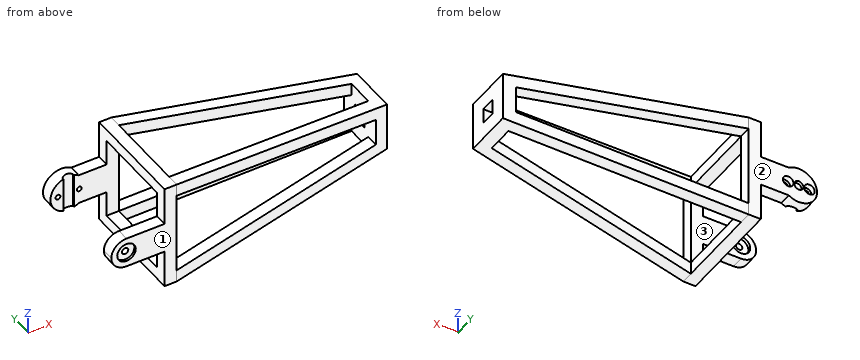
```python
from build123d import *

# Parameters (mm, degrees)
SZKIC1_W                        = 43
SZKIC1_H                        = 20
SZKIC1_R                        = 2.1
DODANIE_WYCI_GNI_CIE1_DEPTH     = 8
SZKIC2_R                        = 6.1
WYTNIJ_WYCI_GNI_CIE1_DEPTH      = 2
WYTNIJ_WYCI_GNI_CIE2_START      = -1.5
SZKIC3_R                        = 6.1
WYTNIJ_WYCI_GNI_CIE2_DEPTH      = 1.5
SZKIC4_W                        = 8
SZKIC4_H                        = 20
DODANIE_WYCI_GNI_CIE2_DEPTH     = 54
ZAOKR_GLENIE1_R                 = 10
DODANIE_WYCI_GNI_CIE3_DEPTH     = 8
WYTNIJ_WYCI_GNI_CIE3_REACH      = 80.313
SZKIC6_R                        = 1.6
SZKIC7_R                        = 3.5
WYTNIJ_WYCI_GNI_CIE4_DEPTH      = 3.5
WYTNIJ_WYCI_GNI_CIE5_REACH      = 83.025
WYTNIJ_WYCI_GNI_CIE5_END_RADIUS = 12
SZKIC10_R                       = 3
WYTNIJ_WYCI_GNI_CIE6_DEPTH      = 2
SZKIC13_W                       = 25
SZKIC13_H                       = 70
DODANIE_WYCI_GNI_CIE4_DEPTH     = 8
WYTNIJ_WYCI_GNI_CIE7_REACH      = 88.568
SZKIC14_W                       = 54
SZKIC14_H                       = 54
DODANIE_WYCI_GNI_CIE5_DEPTH     = 70
WYTNIJ_WYCI_GNI_CIE9_DEPTH      = 209.060087508
WYTNIJ_WYCI_GNI_CIE10_REACH     = 212.119
SZKIC20_W                       = 10
SZKIC20_H                       = 10


with BuildPart() as part:
    # Szkic1 → Dodanie-wyciągnięcie1 (new body)
    with BuildSketch(Plane(origin=(0, 0, 0), x_dir=(1, 0, 0), z_dir=(0, 1, 0))):
        with Locations((11.5, 0)):
            Rectangle(SZKIC1_W, SZKIC1_H)
        with Locations(Location((0, 0, 0), (0, 0, 270))):
            Circle(SZKIC1_R, mode=Mode.SUBTRACT)
    extrude(amount=DODANIE_WYCI_GNI_CIE1_DEPTH)

    # Szkic2 → Wytnij-wyciągnięcie1 (cut)
    with BuildSketch(Plane(origin=(0, 8, 0), x_dir=(1, 0, 0), z_dir=(0, 1, 0))):
        with Locations(Location((0, 0, 0), (0, 0, 270))):
            Circle(SZKIC2_R)
    extrude(amount=-WYTNIJ_WYCI_GNI_CIE1_DEPTH, mode=Mode.SUBTRACT)

    # Szkic3 → Wytnij-wyciągnięcie2 (cut)
    with BuildSketch(Plane.XZ.offset(WYTNIJ_WYCI_GNI_CIE2_START)):
        with Locations(Location((0, 0, 0), (0, 0, 90))):
            Circle(SZKIC3_R)
    extrude(amount=WYTNIJ_WYCI_GNI_CIE2_DEPTH, mode=Mode.SUBTRACT)

    # Szkic4 → Dodanie-wyciągnięcie2 (add)
    with BuildSketch(Plane(origin=(0, 8, 0), x_dir=(1, 0, 0), z_dir=(0, 1, 0))):
        with Locations((29, 0)):
            Rectangle(SZKIC4_W, SZKIC4_H)
    extrude(amount=DODANIE_WYCI_GNI_CIE2_DEPTH)

    # Zaokrąglenie1
    zaokr_glenie1_edges = [part.edges().sort_by_distance(p)[0] for p in [
        (-10, 4, -10),
        (-10, 4, 10),
    ]]
    fillet(zaokr_glenie1_edges, radius=ZAOKR_GLENIE1_R - 0.0001)  # a hair under: the kernel refuses the full size

    # Szkic5 → Dodanie-wyciągnięcie3 (add)
    with BuildSketch(Plane(origin=(0, 62, 0), x_dir=(1, 0, 0), z_dir=(0, 1, 0))):
        with BuildLine():
            Line((33, -10), (33, 10))
            Line((33, 10), (6.633249581, 10))
            ThreePointArc((6.633249581, 10), (-12, 0), (6.633249581, -10))
            Line((6.633249581, -10), (33, -10))
        make_face()
    extrude(amount=DODANIE_WYCI_GNI_CIE3_DEPTH)

    # Szkic6 → Wytnij-wyciągnięcie3 (cut, up to next)
    with BuildSketch(Plane(origin=(0, 70, 0), x_dir=(1, 0, 0), z_dir=(0, 1, 0)), mode=Mode.PRIVATE) as wytnij_wyci_gni_cie3_sk1:
        with Locations(Location((-7, 0, 0), (0, 0, 270))):
            Circle(SZKIC6_R)
    wytnij_wyci_gni_cie3_tool1 = extrude(wytnij_wyci_gni_cie3_sk1.sketch, amount=-WYTNIJ_WYCI_GNI_CIE3_REACH, mode=Mode.PRIVATE) & part.part
    # Szkic6 → Wytnij-wyciągnięcie3 (cut, up to next)
    with BuildSketch(Plane(origin=(0, 70, 0), x_dir=(1, 0, 0), z_dir=(0, 1, 0)), mode=Mode.PRIVATE) as wytnij_wyci_gni_cie3_sk2:
        with Locations(Location((7, 0, 0), (0, 0, 270))):
            Circle(SZKIC6_R)
    wytnij_wyci_gni_cie3_tool2 = extrude(wytnij_wyci_gni_cie3_sk2.sketch, amount=-WYTNIJ_WYCI_GNI_CIE3_REACH, mode=Mode.PRIVATE) & part.part
    add(wytnij_wyci_gni_cie3_tool1.solids().sort_by_distance((-7, 70, 0))[0], mode=Mode.SUBTRACT)
    add(wytnij_wyci_gni_cie3_tool2.solids().sort_by_distance((7, 70, 0))[0], mode=Mode.SUBTRACT)

    # Szkic7 → Wytnij-wyciągnięcie4 (cut)
    with BuildSketch(Plane(origin=(0, 70, 0), x_dir=(1, 0, 0), z_dir=(0, 1, 0))):
        with Locations(Location((7, 0, 0), (0, 0, 270))):
            Circle(SZKIC7_R)
        with Locations(Location((-7, 0, 0), (0, 0, 270))):
            Circle(SZKIC7_R)
    extrude(amount=-WYTNIJ_WYCI_GNI_CIE4_DEPTH, mode=Mode.SUBTRACT)

    # Wytnij-wyciągnięcie5: up to this cylinder (the profile starts inside it)
    wytnij_wyci_gni_cie5_end = Plane(origin=(0, 63.035303, 0), z_dir=(0, -1, 0)) * Cylinder(WYTNIJ_WYCI_GNI_CIE5_END_RADIUS, 191.05, mode=Mode.PRIVATE)
    # Szkic9 → Wytnij-wyciągnięcie5 (cut, up to the surface)
    with BuildSketch(Plane.XY.offset(12), mode=Mode.PRIVATE) as wytnij_wyci_gni_cie5_sk1:
        with BuildLine():
            Line((-3.5, 62), (3.5, 62))
            Line((3.5, 62), (3.5, 63))
            ThreePointArc((3.5, 63), (0, 64.429285786), (-3.5, 63))
            Line((-3.5, 63), (-3.5, 62))
        make_face()
    wytnij_wyci_gni_cie5_tool1 = extrude(wytnij_wyci_gni_cie5_sk1.sketch, amount=-WYTNIJ_WYCI_GNI_CIE5_REACH, mode=Mode.PRIVATE) & wytnij_wyci_gni_cie5_end
    add(wytnij_wyci_gni_cie5_tool1.solids().sort_by_distance((0, 63.035303, 12))[0], mode=Mode.SUBTRACT)

    # Szkic10 → Wytnij-wyciągnięcie6 (cut)
    with BuildSketch(Plane(origin=(0, 70, 0), x_dir=(1, 0, 0), z_dir=(0, 1, 0))):
        with Locations(Location((0, 0, 0), (0, 0, 270))):
            Circle(SZKIC10_R)
    extrude(amount=-WYTNIJ_WYCI_GNI_CIE6_DEPTH, mode=Mode.SUBTRACT)

    # Szkic13 → Dodanie-wyciągnięcie4 (add)
    with BuildSketch(Plane(origin=(33, 0, 0), x_dir=(0, 0, -1), z_dir=(1, 0, 0))):
        with Locations((22.5, 35)):
            Rectangle(SZKIC13_W, SZKIC13_H)
        with Locations((-22.5, 35)):
            Rectangle(SZKIC13_W, SZKIC13_H)
    extrude(amount=-DODANIE_WYCI_GNI_CIE4_DEPTH)

    # Szkic14 → Wytnij-wyciągnięcie7 (cut, up to next)
    with BuildSketch(Plane.ZY.offset(-25), mode=Mode.PRIVATE) as wytnij_wyci_gni_cie7_sk1:
        with Locations((0, 35)):
            Rectangle(SZKIC14_W, SZKIC14_H)
    wytnij_wyci_gni_cie7_tool1 = extrude(wytnij_wyci_gni_cie7_sk1.sketch, amount=-WYTNIJ_WYCI_GNI_CIE7_REACH, mode=Mode.PRIVATE) & part.part
    add(wytnij_wyci_gni_cie7_tool1.solids().sort_by_distance((25, 35, 0))[0], mode=Mode.SUBTRACT)

    # Szkic17 → Dodanie-wyciągnięcie5 (add, through all)
    with BuildSketch(Plane.XZ):
        Polygon((33, 35), (183, 16), (183, -16), (33, -35), (33, -26.936077602), (175, -8.949410935), (175, 8.949410935), (33, 26.936077602), align=None)
    extrude(amount=-DODANIE_WYCI_GNI_CIE5_DEPTH)

    # Szkic18 → Wytnij-wyciągnięcie9 (cut, through all)
    with BuildSketch(Plane(origin=(0, 0, -35), x_dir=(-1, 0, 0), z_dir=(0, 0, -1))):
        Polygon((-33, 70), (-183, 70), (-183, 51), align=None)
        Polygon((-183, 0), (-183, 19), (-33, 0), align=None)
        Polygon((-33, 8.063922398), (-33, 61.936077602), (-175, 43.949410935), (-175, 26.050589065), align=None)
    extrude(amount=-WYTNIJ_WYCI_GNI_CIE9_DEPTH, mode=Mode.SUBTRACT)

    # Szkic20 → Wytnij-wyciągnięcie10 (cut, up to next)
    with BuildSketch(Plane(origin=(183, 0, 0), x_dir=(0, 0, -1), z_dir=(1, 0, 0)), mode=Mode.PRIVATE) as wytnij_wyci_gni_cie10_sk1:
        with Locations((0, 35)):
            Rectangle(SZKIC20_W, SZKIC20_H)
    wytnij_wyci_gni_cie10_tool1 = extrude(wytnij_wyci_gni_cie10_sk1.sketch, amount=-WYTNIJ_WYCI_GNI_CIE10_REACH, mode=Mode.PRIVATE) & part.part
    add(wytnij_wyci_gni_cie10_tool1.solids().sort_by_distance((183, 35, 0))[0], mode=Mode.SUBTRACT)


solid = part.part
```
The model under review builds one solid part; all positions refer to its coordinate system, in mm. Face numbers are marked on the shaded views. Give positions to 0.01 mm unless a question says otherwise; leave off trailing zeros. Loops run counter-clockwise (first coordinate to the right, second up) from the corner with the lowest first, then second, coordinate; pieces in that order, holes last. Notation, with made-up numbers: (55, 37.5) - (79, 37.5) arc R31 cw to (79, 69.5) - close; hole circle Ø2 at (-12, 1). An arc over 180 degrees is marked (long way). Answer as a JSON object with one key per item and string values.
Q1. To check wall thickness, follow line 1 along X through (y, z) = (63, 0); line 2 along Y through (x, z) = (15, 9); line 3 along X through (y, z) = (3.85, 0). State the ranges of each line that lie inside material, in increasing order.
Worked out:
{"line 1": "x = -12 to -8.6, -5.4 to -3.5, 3.5 to 5.4, 8.6 to 33", "line 2": "y = 0 to 8, 62 to 70", "line 3": "x = -10 to -2.1, 2.1 to 33"}
Q2. Add section B-B on x = 96. State the section outline as (y, z) points.
Worked out:
{"outline": "(7.98, -27.02) - (16.04, -27.02) - (16.04, -18.96) - (7.98, -18.96) - close; (7.98, 18.96) - (16.04, 18.96) - (16.04, 27.02) - (7.98, 27.02) - close; (53.96, -27.02) - (62.02, -27.02) - (62.02, -18.96) - (53.96, -18.96) - close; (53.96, 18.96) - (62.02, 18.96) - (62.02, 27.02) - (53.96, 27.02) - close"}
Q3. Insertion check: pin 1 (4 mm diameter, centred on x = 16, y = 4, fed in from -Z); pin 2 (5 mm diameter, centred on x = 0, z = 0, fed in from -Y); pin 3 (2 mm diameter, centred on y = 45, z = 22, fed in from -X); pin 4 (4 mm diameter, centred on y = 66.5, z = 7, fed in from +X). Each pin has a flat end and moves straight along its axis. Give the tip position at first contact, or say it passes through.
Worked out:
{"pin 1": "stops at z = -10", "pin 2": "stops at y = 1.5", "pin 3": "passes through", "pin 4": "stops at x = 33"}
Q4. Mouldability with a two-part tool opening along Y and no side actions: class the marked faces 1, 2 and 3 as +Y half, -Y half, draft (parallel to the pull), parting line (faces both ways), or undercut.
Worked out:
{"face 1": "-Y half", "face 2": "+Y half", "face 3": "undercut"}
Q5. Add section A-A on x = 28. State the section outline as (y, z) points.
Worked out:
{"outline": "(0, -35) - (70, -35) - (70, 35) - (0, 35) - close; hole (8, -27) - (62, -27) - (62, 27) - (8, 27) - close"}
